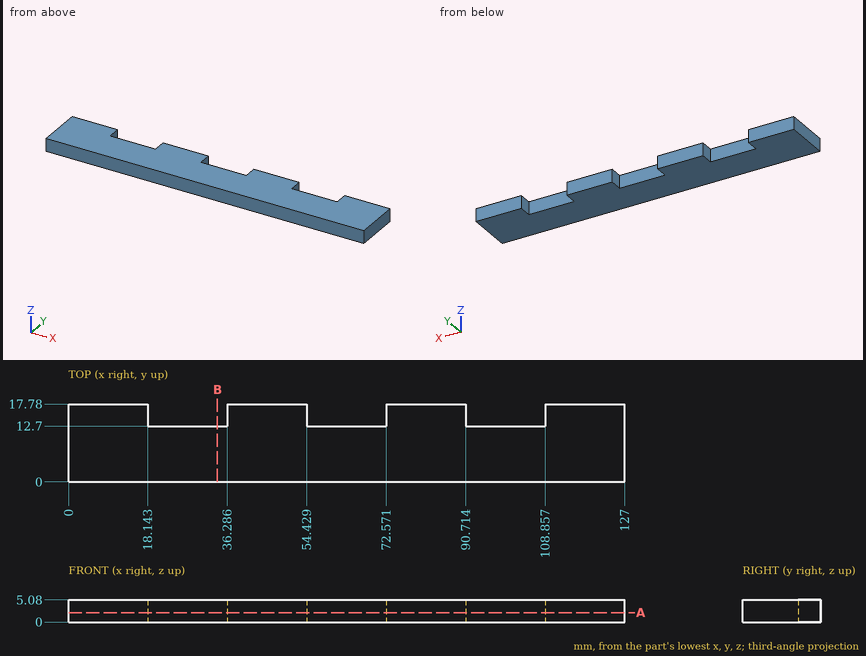
Design review of the part shown in the three views and the two pictorial views. Dimensions are in mm from the part's minimum x, y and z. Round coordinates to 2 decimals unless told otherwise and drop trailing zeros. Write each loop counter-clockwise with the first axis right and the second up, starting at its lowest first coordinate (ties: lowest second). Pieces come first, ordered by that corner, then holes. Notation, with made-up numbers: M 12.25,-25 L 24.25,-25 A29 cw 24.25,14 Z; hole C 57,60 d8. An arc over 180 degrees is marked long. One line per item, written item: value. Start each with the question number.
1. Clearance check with a flat-ended pin moving along its axis: P1, Ø1.5, axis at x = 67, z = 2.5, coming from the +Y side. State where the tip first meets the part, or that it passes through.
2. Take a section at B-B on x = 34. State the section outline as (y, z) points, then the cut area to 3 significant figures.
3. Take a section at A-A on z = 2.15. State the section outline as (x, y) points (1 decimal), then the cut area to 3 significant figures.
4. To check wall thickness, follow probe 1 along X at (y, z) = (13.75, 2.4) (1 decimal); probe 2 along Y at (x, z) = (56.5, 4.05). State the ranges of each line that lie inside material, in increasing order. Write a range as from..to.
Computed:
1. P1: stops at y = 12.7
2. outline: M 0,0 L 12.7,0 L 12.7,5.08 L 0,5.08 Z
2. area: 64.5 mm²
3. outline: M 0,0 L 127,0 L 127,17.8 L 108.9,17.8 L 108.9,12.7 L 90.7,12.7 L 90.7,17.8 L 72.6,17.8 L 72.6,12.7 L 54.4,12.7 L 54.4,17.8 L 36.3,17.8 L 36.3,12.7 L 18.1,12.7 L 18.1,17.8 L 0,17.8 Z
3. area: 1,980 mm²
4. probe 1: x = 0..18.1, 36.3..54.4, 72.6..90.7, 108.9..127
4. probe 2: y = 0..12.7
